Autodesk Inventor part; units mm, degrees
ref_plane "YZ Plane" through (0, 0, 0) normal (1, 0, 0) x (0, 1, 0)
ref_plane "XZ Plane" through (0, 0, 0) normal (0, 1, 0) x (-1, 0, 0)
ref_plane "XY Plane" through (0, 0, 0) normal (0, 0, 1) x (1, 0, 0)
sketch "Esboço1" plane through (0, 0, 0) normal (1, 0, 0) x (0, 1, 0)
  circle A0 centre (0, 0) radius 10
  dimension "d0" = 20
extrude "Extrusão1" add sketch "Esboço1" along normal blind 8
sketch "Esboço2" plane through (8, 0, 0) normal (1, 0, 0) x (0, 0, -1)
  circle A0 centre (0, 0) radius 2
  dimension "d3" = 4
extrude "Extrusão2" cut sketch "Esboço2" against normal blind 2
sketch "Esboço3" plane through (6, 0, 0) normal (1, 0, 0) x (0, 0, -1)
  line L0 (1, 0) -> (1, 1.7321)
  circle A0 centre (0, 0) radius 2
  line L1 (1, 0) -> (1, -1.7321)
  line L2 (-1, 0) -> (-1, 1.7321)
  line L3 (-1, 0) -> (-1, -1.7321)
  arc A1 (-1, 1.7321) -> (0, 2) centre (0, 0) ccw
  arc A2 (-1, -1.7321) -> (1, -1.7321) centre (0, 0) ccw
  dimension "d6" = 1
  dimension "d7" = 1
extrude "Extrusão3" cut sketch "Esboço3" against normal through all contours L1 A0 L3 L2 L0
sketch "Esboço4" plane through (8, 0, 0) normal (1, 0, 0) x (0, 0, -1)
  circle A0 centre (0, 0) radius 2
  circle A1 centre (0, 0) radius 11
  dimension "d10" = 22
extrude "Extrusão4" add sketch "Esboço4" against normal blind 1
sketch "Esboço5" plane through (0, 0, 0) normal (-1, 0, 0) x (0, 0, 1)
  circle A0 centre (0, 0) radius 2
  circle A1 centre (0, 0) radius 11
extrude "Extrusão5" add sketch "Esboço5" against normal blind 1
properties part number "RODA MOTOR-PASSO"
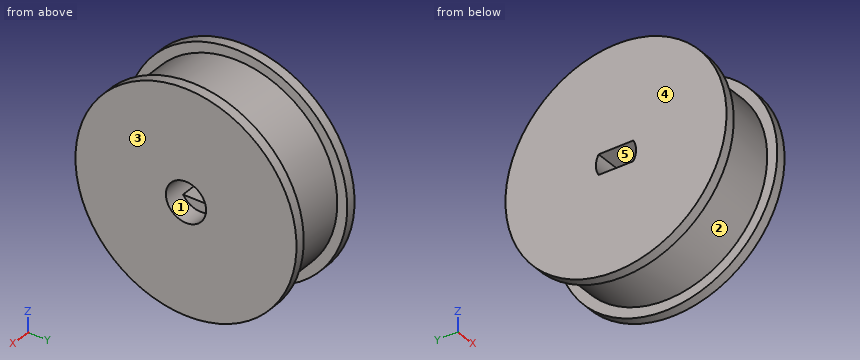
Verification items for the finished model (mm, model axes). Face numbers are marked on the shaded views. A direction names the side the tool comes from. Coordinates: 2 decimals unless noted, no trailing zeros. Order: outer loops, then holes, each group sorted by start corner. A loop starts at its lowest first (then second) coordinate and runs counter-clockwise, first axis right, second up. Notation, with made-up numbers: M -17.5,-35.75 L 4.5,-35.75 A33 cw 4.5,-4.75 Z; hole C 36.5,45.5 d5. An arc over 180 degrees is marked long. Return JSON: item names as keys, results as strings.
1) Thickness scan on L1, parallel to Y at x = 6, z = 0; L2, parallel to Z at x = 3.25, y = 0; L3, parallel to Z at x = 2, y = 1.25. Record the ranges inside material, lowest first. Write a range as [from, to].
Answer list:
{"L1": "[-10, -2], [2, 10]", "L2": "[-10, -1], [1, 10]", "L3": "[-9.92, -1], [1, 9.92]"}
2) Access from +Z, -Z, +X, -X, +Y, -Y to the whole of each face (thin tool, end or side, straight path). Record for the marked faces 4 and 5.
Answer list:
{"face 4": "+Z, -Z, -X, +Y, -Y", "face 5": "+X, -X"}
3) Cross-section at B-B, the plane z = 0. Record the boundary of the cut face in (x, y), and give its area (3 significant figures).
Answer list:
{"outline": "M 0,-11 L 1,-11 L 1,-10 L 7,-10 L 7,-11 L 8,-11 L 8,-2 L 0,-2 Z; M 0,2 L 8,2 L 8,11 L 7,11 L 7,10 L 1,10 L 1,11 L 0,11 Z", "area": "132 mm2"}
4) Cross-section at D-D, the plane y = 2.5. Record the boundary of the cut face in (x, z).
Answer list:
{"outline": "M 0,-10.71 L 1,-10.71 L 1,-9.68 L 7,-9.68 L 7,-10.71 L 8,-10.71 L 8,10.71 L 7,10.71 L 7,9.68 L 1,9.68 L 1,10.71 L 0,10.71 Z"}
5) Cross-section at C-C, the plane z = 3.5. Record the boundary of the cut face in (x, y).
Answer list:
{"outline": "M 0,-10.43 L 1,-10.43 L 1,-9.37 L 7,-9.37 L 7,-10.43 L 8,-10.43 L 8,10.43 L 7,10.43 L 7,9.37 L 1,9.37 L 1,10.43 L 0,10.43 Z"}
6) Cross-section at A-A, the plane y = 0. Record the boundary of the cut face in (x, z).
Answer list:
{"outline": "M 0,-11 L 1,-11 L 1,-10 L 7,-10 L 7,-11 L 8,-11 L 8,-2 L 6,-2 L 6,-1 L 0,-1 Z; M 0,1 L 6,1 L 6,2 L 8,2 L 8,11 L 7,11 L 7,10 L 1,10 L 1,11 L 0,11 Z"}
7) Release check for a two-part mould opening along Y. For the marked faces 1, 2 and 3 record: +Y half, -Y half, draft (parallel to the pull), parting line (faces both ways), or undercut.
Answer list:
{"face 1": "undercut", "face 2": "parting line", "face 3": "draft"}
8) Gauge pin test, flat ends, axial feed: pin 1 (0.5 mm diameter, centred on y = 0.5, z = -1.5, fed in from +X); pin 2 (1.5 mm diameter, centred on x = 6.5, y = -5.5, fed in from +Z); pin 3 (1 mm diameter, centred on x = 3, y = 0.5, fed in from +Z); pin 4 (10 mm diameter, centred on y = 5.5, z = 7, fed in from -X). Record the tip position at first contact, or that the pin passes through.
Answer list:
{"pin 1": "x = 6", "pin 2": "z = 9.83", "pin 3": "z = 10", "pin 4": "x = 0"}
